from build123d import *

# Parameters (mm, degrees)
F0_R     = 100
F0_R_2   = 27.5
F1_DEPTH = 4
F2_R     = 40
F2_R_2   = 27.5
F3_DEPTH = 57
F4_R     = 100
F4_R_2   = 27.5
F5_DEPTH = 4
F7_DEPTH = 30
F9_DEPTH = 30


with BuildPart() as f1:
    # F0 (on Front) → F1 (new body)
    with BuildSketch(Plane.XZ):
        Circle(F0_R)
        Circle(F0_R_2, mode=Mode.SUBTRACT)
    extrude(amount=F1_DEPTH)

    # F2 (on face) → F3 (join)
    with BuildSketch(Plane.XZ.offset(4)):
        Circle(F2_R)
        Circle(F2_R_2, mode=Mode.SUBTRACT)
    extrude(amount=F3_DEPTH)

    # F4 (on face) → F5 (join)
    with BuildSketch(Plane.XZ.offset(61)):
        Circle(F4_R)
        Circle(F4_R_2, mode=Mode.SUBTRACT)
    extrude(amount=F5_DEPTH)

    # F6 (on face) → F7 (cut)
    with BuildSketch(Plane(origin=(0, 0, 0), x_dir=(-1, 0, 0), z_dir=(0, 1, 0))):
        with BuildLine():
            ThreePointArc((32.408965, 19.866025), (19.006578, 32.920358), (1, 38))
            Line((1, 38), (1, 29.483046))
            ThreePointArc((1, 29.483046), (14.75, 25.547749), (25.033067, 15.607548))
            Line((25.033067, 15.607548), (32.408965, 19.866025))
        make_face()
        with BuildLine():
            ThreePointArc((-25.033067, 15.607548), (-14.75, 25.547749), (-1, 29.483046))
            Line((-1, 29.483046), (-1, 38))
            ThreePointArc((-1, 38), (-19.006578, 32.920358), (-32.408965, 19.866025))
            Line((-32.408965, 19.866025), (-25.033067, 15.607548))
        make_face()
        with BuildLine():
            ThreePointArc((-26.033067, -13.875498), (-29.5, 0), (-26.033067, 13.875498))
            Line((-26.033067, 13.875498), (-33.408965, 18.133975))
            ThreePointArc((-33.408965, 18.133975), (-38.013156, 0), (-33.408965, -18.133975))
            Line((-33.408965, -18.133975), (-26.033067, -13.875498))
        make_face()
        with BuildLine():
            ThreePointArc((-1, -29.483046), (-14.75, -25.547749), (-25.033067, -15.607548))
            Line((-25.033067, -15.607548), (-32.408965, -19.866025))
            ThreePointArc((-32.408965, -19.866025), (-19.006578, -32.920358), (-1, -38))
            Line((-1, -38), (-1, -29.483046))
        make_face()
        with BuildLine():
            ThreePointArc((25.033067, -15.607548), (14.75, -25.547749), (1, -29.483046))
            Line((1, -29.483046), (1, -38))
            ThreePointArc((1, -38), (19.006578, -32.920358), (32.408965, -19.866025))
            Line((32.408965, -19.866025), (25.033067, -15.607548))
        make_face()
        with BuildLine():
            ThreePointArc((26.033067, 13.875498), (29.5, 0), (26.033067, -13.875498))
            Line((26.033067, -13.875498), (33.408965, -18.133975))
            ThreePointArc((33.408965, -18.133975), (38.013156, 0), (33.408965, 18.133975))
            Line((33.408965, 18.133975), (26.033067, 13.875498))
        make_face()
    extrude(amount=-F7_DEPTH, mode=Mode.SUBTRACT)

    # F8 (on face) → F9 (cut)
    with BuildSketch(Plane.XZ.offset(65)):
        with BuildLine():
            ThreePointArc((32.408965, 19.866025), (19.006578, 32.920358), (1, 38))
            Line((1, 38), (1, 29.483046))
            ThreePointArc((1, 29.483046), (14.75, 25.547749), (25.033067, 15.607548))
            Line((25.033067, 15.607548), (32.408965, 19.866025))
        make_face()
        with BuildLine():
            Line((-32.408965, 19.866025), (-25.033067, 15.607548))
            ThreePointArc((-25.033067, 15.607548), (-14.75, 25.547749), (-1, 29.483046))
            Line((-1, 29.483046), (-1, 38))
            ThreePointArc((-1, 38), (-19.006578, 32.920358), (-32.408965, 19.866025))
        make_face()
        with BuildLine():
            Line((-33.408965, -18.133975), (-26.033067, -13.875498))
            ThreePointArc((-26.033067, -13.875498), (-29.5, 0), (-26.033067, 13.875498))
            Line((-26.033067, 13.875498), (-33.408965, 18.133975))
            ThreePointArc((-33.408965, 18.133975), (-38.013156, 0), (-33.408965, -18.133975))
        make_face()
        with BuildLine():
            Line((-1, -38), (-1, -29.483046))
            ThreePointArc((-1, -29.483046), (-14.75, -25.547749), (-25.033067, -15.607548))
            Line((-25.033067, -15.607548), (-32.408965, -19.866025))
            ThreePointArc((-32.408965, -19.866025), (-19.006578, -32.920358), (-1, -38))
        make_face()
        with BuildLine():
            Line((32.408965, -19.866025), (25.033067, -15.607548))
            ThreePointArc((25.033067, -15.607548), (14.75, -25.547749), (1, -29.483046))
            Line((1, -29.483046), (1, -38))
            ThreePointArc((1, -38), (19.006578, -32.920358), (32.408965, -19.866025))
        make_face()
        with BuildLine():
            Line((33.408965, 18.133975), (26.033067, 13.875498))
            ThreePointArc((26.033067, 13.875498), (29.5, 0), (26.033067, -13.875498))
            Line((26.033067, -13.875498), (33.408965, -18.133975))
            ThreePointArc((33.408965, -18.133975), (38.013156, 0), (33.408965, 18.133975))
        make_face()
    extrude(amount=-F9_DEPTH, mode=Mode.SUBTRACT)


solid = f1.part
Here's how the part is built. I have some questions about the finished solid (model axes, mm). A direction names the side the tool comes from. Coordinates: 2 decimals unless noted, no trailing zeros. Order: outer loops, then holes, each group sorted by start corner. A loop starts at its lowest first (then second) coordinate and runs counter-clockwise, first axis right, second up. Notation, with made-up numbers: (24.5, 51.25) -> (36.5, 51.25) arc R20 cw to (36.5, 63.25) -> close; hole circle Ø11 at (-10, 37.5). An arc over 180 degrees is marked (long way). Answer in a Markdown table with one row per item.
(1) I want a section at A-A on y = -47.5. List the corners of the cut face in (x, z) for me, then the cut area to 3 significant figures.
Answer key:
| item | result |
|---|---|
| outline | circle Ø80 at (0, 0); hole (-33.41, -18.13) -> (-26.03, -13.88) arc R29.5 cw to (-26.03, 13.88) -> (-33.41, 18.13) arc R38.01 ccw to start; hole (-32.41, -19.87) arc R38.01 ccw to (-1, -38) -> (-1, -29.48) arc R29.5 cw to (-25.03, -15.61) -> close; hole (-32.41, 19.87) -> (-25.03, 15.61) arc R29.5 cw to (-1, 29.48) -> (-1, 38) arc R38.01 ccw to start; hole circle Ø55 at (0, 0); hole (1, -38) arc R38.01 ccw to (32.41, -19.87) -> (25.03, -15.61) arc R29.5 cw to (1, -29.48) -> close; hole (1, 29.48) arc R29.5 cw to (25.03, 15.61) -> (32.41, 19.87) arc R38.01 ccw to (1, 38) -> close; hole (26.03, -13.88) -> (33.41, -18.13) arc R38.01 ccw to (33.41, 18.13) -> (26.03, 13.88) arc R29.5 cw to start |
| area | 947 mm^2 |
(2) Thinking about a two-plate mould opening in Z: for faces 1 (the face through (-1, -61, -43)), 2 (the face through (38.012, -14.79, 0.265)), 3 (the face through (95.38, -62.97, 30.04)), which applies, +Z half, -Z half, draft (parallel to the pull), parting line (faces both ways), or undercut?
Answer key:
| item | result |
|---|---|
| face 1 | draft |
| face 2 | undercut |
| face 3 | parting line |
(3) Will these pins go through, and if not, where does the flat tip stop? pin 1 Ø7 at (y, z) = (-10.5, -34) entering from -X; pin 2 Ø1.5 at (y, z) = (-23, 20.5) entering from -X; pin 3 Ø7 at (y, z) = (-50, -33) entering from -X.
Answer key:
| item | result |
|---|---|
| pin 1 | x = -25.88 |
| pin 2 | x = -34.78 |
| pin 3 | x = -27.01 |
(4) I want a section at D-D on z = 50. List the corners of the cut face in (x, y) for me.
Answer key:
| item | result |
|---|---|
| outline | (-86.6, -65) -> (86.6, -65) -> (86.6, -61) -> (-86.6, -61) -> close; (-86.6, -4) -> (86.6, -4) -> (86.6, 0) -> (-86.6, 0) -> close |
(5) On a 3-axis mill with a long thin cutter (end or side, diameter ignored), from which of +Z, -Z, +X, -X, +Y, -Y can I reach the whole of each face in a straight line? I mean faces 4 (the face through (28.669, -14.79, -17.707)), 5 (the face through (-8.67, -32.1, -39.05)), 6 (the face through (29.773, -50.21, 16.035)). Say none if no direction works.
Answer key:
| item | result |
|---|---|
| face 4 | +Y |
| face 5 | none |
| face 6 | -Y |
(6) Please list where these lines run through material, in increasing order: probe 1 along Z at (x, y) = (0, -49); probe 2 along X at (y, z) = (-54, 0.5); probe 3 along Y at (x, z) = (-25, -34.5).
Answer key:
| item | result |
|---|---|
| probe 1 | -40 to -27.5, 27.5 to 40 |
| probe 2 | -40 to -38.01, -29.5 to -27.5, 27.5 to 29.5, 38.01 to 40 |
| probe 3 | -65 to -61, -4 to 0 |
